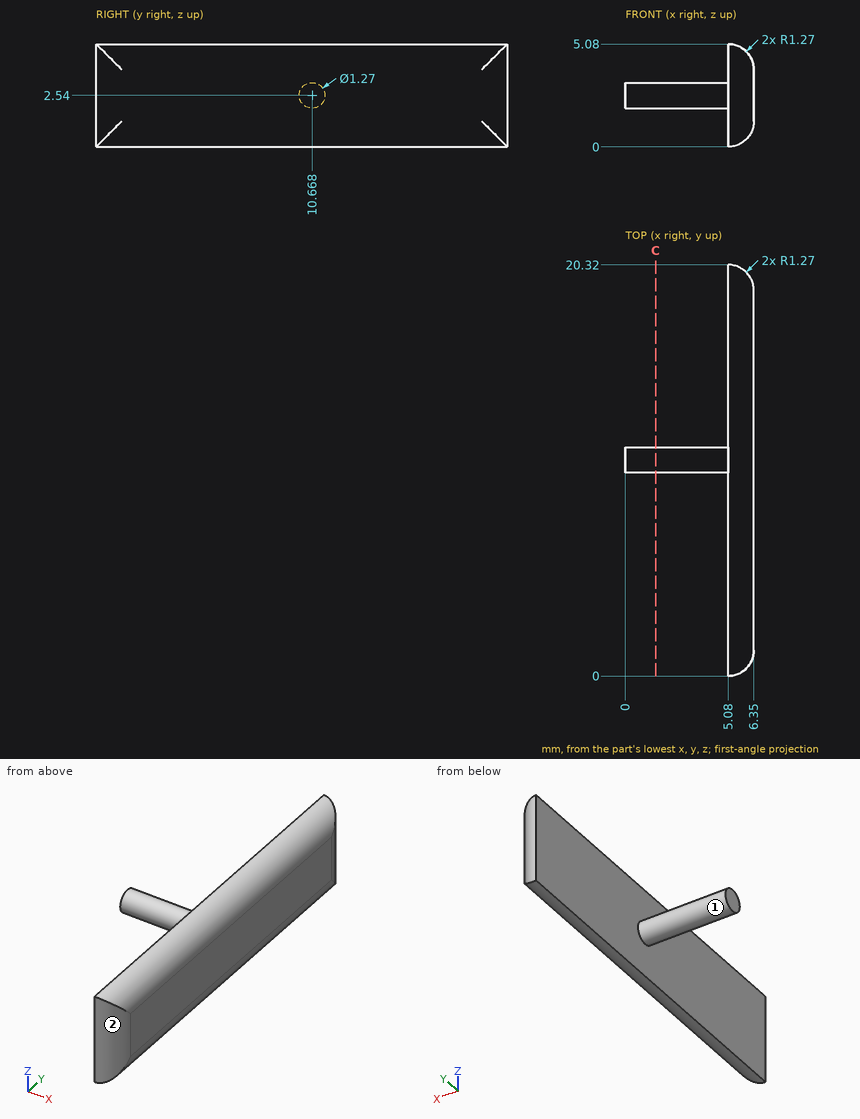
Here's the drawing with two shaded views (mm, measured from the low corner). I have some questions. A direction names the side the tool comes from. Round coordinates to 2 decimals unless told otherwise and drop trailing zeros. Loops run counter-clockwise (first coordinate to the right, second up) from the corner with the lowest first, then second, coordinate; pieces in that order, holes last.
1. For the marked faces 1 and 2, which set-ups out of +Z, -Z, +X, -X, +Y, -Y let a thin tool reach every point of the face, with its end or its side?
Answers:
face 1: -X
face 2: +Z, -Z, +X, -Y
2. Suppose I cut it at C-C, the plane x = 1.5. Please give me the cut outline in (y, z) (3 decimals), and give its area (3 significant figures).
Answers:
outline: circle Ø1.27 at (10.668, 2.54)
area: 1.27 mm2
3. Will these pins go through, and if not, where does the flat tip stop? pin 1 (1.5 mm diameter, centred on y = 14, z = 3.5, fed in from -X); pin 2 (3 mm diameter, centred on x = 3, z = 2, fed in from -Y).
Answers:
pin 1: stops at x = 5.08
pin 2: stops at y = 10.03
4. If I drill on probe 1 along X at (y, z) = (12.75, 3.3); probe 2 along Y at (x, z) = (5, 2.6); probe 3 along Z at (x, y) = (2, 10.75), over which ranges is the centre line in solid material (lowest first)?
Answers:
probe 1: x = 5.08 to 6.35
probe 2: y = 10.04 to 11.3
probe 3: z = 1.91 to 3.17
